The model under review builds one solid part; all positions refer to its coordinate system, in mm. Give positions to 0.01 mm unless a question says otherwise; leave off trailing zeros. Order: outer loops, then holes, each group sorted by start corner. A loop starts at its lowest first (then second) coordinate and runs counter-clockwise, first axis right, second up. Notation, with made-up numbers: M 66.5,-6.75 L 84.5,-6.75 A14 cw 84.5,6.25 Z; hole C -4.75,-25.75 d5. An arc over 180 degrees is marked long. One line per question, with ' | ' between items. Start each with the question number.
1. The part is to be moulded in two halves that separate along Z. For faces 1 (the face through (-0.493, -1.802, -5.723)), 2 (the face through (0, 4, 5)), 3 (the face through (-8.4, 7.81, 1.73)), say which applies: +Z half, -Z half, draft (parallel to the pull), parting line (faces both ways), or undercut.
2. We need section A-A on y = 0. Write out the cut boundary in (x, z), then the cut area to 3 significant figures.
3. Insertion check: P1, Ø8, axis at x = -5, y = 5, coming from the -Z side; P2, Ø1.5, axis at y = 0, z = 4, coming from the -X side; P3, Ø2, axis at x = -12, z = 1.5, coming from the +Y side; P4, Ø1, axis at x = -4.5, y = -3, coming from the -Z side. Each pin has a flat end and moves straight along its axis. Give the tip position at first contact, or say it passes through.
4. We need section C-C on x = -14. Write out the cut boundary in (y, z).
5. Wall thickness on L1, parallel to Y at x = -0.4, z = 0; L2, parallel to Y at x = -16.5, z = 0; L3, parallel to Z at x = -15, y = 0.75: over which ranges is each line inside the solid? List them lowest first.
```python
from build123d import *

# Parameters (mm, degrees)
CHAFL_N10_SIZE = 0.25


with BuildPart() as part:
    # Sketch1 → Revolve1 (revolve)
    with BuildSketch(Plane.XY, mode=Mode.PRIVATE) as revolve1_sk:
        Polygon((-17.979823496, 7.383932563), (-17.031162834, 8), (0, 8), (0, 6), (-0.979823496, 6), (-0.979823496, 6.888071888), (-17.979823496, 6.888071888), align=None)
    revolve(revolve1_sk.sketch.rotate(Axis((0, 0, 0), (-1, 0, 0)), 90), axis=Axis((0, 0, 0), (-1, 0, 0)))

    # Chaflán10
    chafl_n10_edges = [part.edges().sort_by_distance(p)[0] for p in [
        (-0.979823496, 0, 6),
        (-17.979823496, 0, 6.888071888),
        (0, 0, 6),
    ]]
    chamfer(chafl_n10_edges, length=CHAFL_N10_SIZE)


solid = part.part
```
Entries:
1) face 1: undercut | face 2: draft | face 3: parting line
2) outline: M -17.98,-7.38 L -17.03,-8 L 0,-8 L 0,-6.25 L -0.25,-6 L -0.73,-6 L -0.98,-6.25 L -0.98,-6.89 L -17.73,-6.89 L -17.98,-7.14 Z; M -17.98,7.14 L -17.73,6.89 L -0.98,6.89 L -0.98,6.25 L -0.73,6 L -0.25,6 L 0,6.25 L 0,8 L -17.03,8 L -17.98,7.38 Z | area: 41.0 mm^2
3) P1: stops at z = -7.94 | P2: passes through | P3: stops at y = 7.98 | P4: stops at z = -7.6
4) outline: C 0,0 d16; hole C 0,0 d13.78
5) L1: y = -8 to -6, 6 to 8 | L2: y = -8 to -6.89, 6.89 to 8 | L3: z = -7.96 to -6.85, 6.85 to 7.96
